Work out the finished part from the listing and answer in its coordinate system (mm). Face numbers are marked on the shaded views. A direction names the side the tool comes from. Round coordinates to 2 decimals unless told otherwise and drop trailing zeros. Order: outer loops, then holes, each group sorted by start corner. A loop starts at its lowest first (then second) coordinate and runs counter-clockwise, first axis right, second up. Notation, with made-up numbers: (63.5, 59.5) -> (112.5, 59.5) arc R24 cw to (112.5, 82.5) -> close; hole circle Ø4 at (33, 12.5). An arc over 180 degrees is marked (long way). Use one line per item in the form item = value.
```python
from build123d import *

# Parameters (mm, degrees)
SKETCH1_W           = 406.4
SKETCH1_H           = 25.4
BOSS_EXTRUDE1_DEPTH = 2.38125
SKETCH2_W           = 406.4
SKETCH2_H           = 25.4
SKETCH2_R           = 6.35
SKETCH2_R_2         = 2.5796875
BOSS_EXTRUDE2_DEPTH = 2.38125
FILLET1_R           = 2.38125


with BuildPart() as part:
    # Sketch1 → Boss-Extrude1 (new body)
    with BuildSketch(Plane(origin=(0, 0, 0), x_dir=(1, 0, 0), z_dir=(0, 1, 0))):
        with Locations((203.2, 12.7)):
            Rectangle(SKETCH1_W, SKETCH1_H)
    extrude(amount=BOSS_EXTRUDE1_DEPTH)

    # Sketch2 → Boss-Extrude2 (add)
    with BuildSketch(Plane.XY):
        with Locations((203.2, 12.7)):
            Rectangle(SKETCH2_W, SKETCH2_H)
        with Locations(Location((12.7, 12.7, 0), (0, 0, 180))):
            Circle(SKETCH2_R, mode=Mode.SUBTRACT)
        with Locations(Location((139.7, 12.7, 0), (0, 0, 180))):
            Circle(SKETCH2_R, mode=Mode.SUBTRACT)
        with Locations(Location((266.7, 12.7, 0), (0, 0, 180))):
            Circle(SKETCH2_R, mode=Mode.SUBTRACT)
        with Locations(Location((393.7, 12.7, 0), (0, 0, 180))):
            Circle(SKETCH2_R, mode=Mode.SUBTRACT)
        with Locations(Location((76.2, 12.7, 0), (0, 0, 180))):
            Circle(SKETCH2_R_2, mode=Mode.SUBTRACT)
        with Locations(Location((203.2, 12.7, 0), (0, 0, 180))):
            Circle(SKETCH2_R_2, mode=Mode.SUBTRACT)
        with Locations(Location((330.2, 12.7, 0), (0, 0, 180))):
            Circle(SKETCH2_R_2, mode=Mode.SUBTRACT)
    extrude(amount=BOSS_EXTRUDE2_DEPTH)

    # Fillet1
    fillet1_edges = [part.edges().sort_by_distance(p)[0] for p in [
        (203.2, 0, 2.38125),
    ]]
    fillet(fillet1_edges, radius=FILLET1_R)


solid = part.part
```
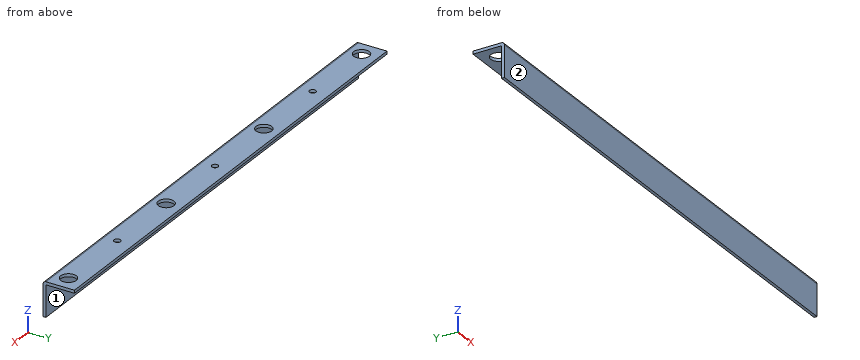
Item 1: Flat-ended cylindrical pins translate along their axes: P1, Ø7, axis at x = 273, y = 13.5, coming from the -Z side; P2, Ø6, axis at x = 268.5, z = -5, coming from the +Y side. Find the tip coordinate at first contact, or state that the pin passes through.
Findings:
P1 = 0
P2 = 2.38
Item 2: For the marked faces 1 and 2, determine the directions among +Z, -Z, +X, -X, +Y, -Y from which every point of the face is accessible in a straight line to the end or side of a thin tool.
Findings:
face_1 = -Z, +X, -X, +Y
face_2 = +Z, -Z, +X, -X, -Y
Item 3: Consider line 1 along Z through (x, y) = (110, 5.25); line 2 along Y through (x, z) = (139.7, 0.85). Determine where each line is inside the solid, lowest interval first.
Findings:
line_1 = 0 to 2.38
line_2 = 0.16 to 6.35, 19.05 to 25.4
Item 4: The part is cut by section C-C, the plane z = -11.5. Give the vertices of the cut face in (x, y), and give its area (3 significant figures).
Findings:
outline = (0, 0) -> (406.4, 0) -> (406.4, 2.38) -> (0, 2.38) -> close
area = 968 mm^2
Item 5: The part is cut by section B-B, the plane x = 210. Give the vertices of the cut face in (y, z), and give its area (3 significant figures).
Findings:
outline = (0, -25.4) -> (2.38, -25.4) -> (2.38, 0) -> (25.4, 0) -> (25.4, 2.38) -> (2.38, 2.38) arc R2.38 ccw to (0, 0) -> close
area = 120 mm^2
Item 6: The part is cut by section A-A, the plane x = 139.7. Give the vertices of the cut face in (y, z), and give its area (3 significant figures).
Findings:
outline = (0, -25.4) -> (2.38, -25.4) -> (2.38, 0) -> (6.35, 0) -> (6.35, 2.38) -> (2.38, 2.38) arc R2.38 ccw to (0, 0) -> close; (19.05, 0) -> (25.4, 0) -> (25.4, 2.38) -> (19.05, 2.38) -> close
area = 89.5 mm^2
